The model under review builds one solid part; all positions refer to its coordinate system, in mm. Face numbers are marked on the shaded views. A direction names the side the tool comes from. Give positions to 0.01 mm unless a question says otherwise; leave off trailing zeros. Loops run counter-clockwise (first coordinate to the right, second up) from the corner with the lowest first, then second, coordinate; pieces in that order, holes last. Notation, with made-up numbers: (47, 54.25) - (91, 54.25) arc R20 cw to (91, 59.25) - close; hole circle Ø6 at (85, 5.5). An arc over 180 degrees is marked (long way). Answer as a JSON object with one key per item and string values.
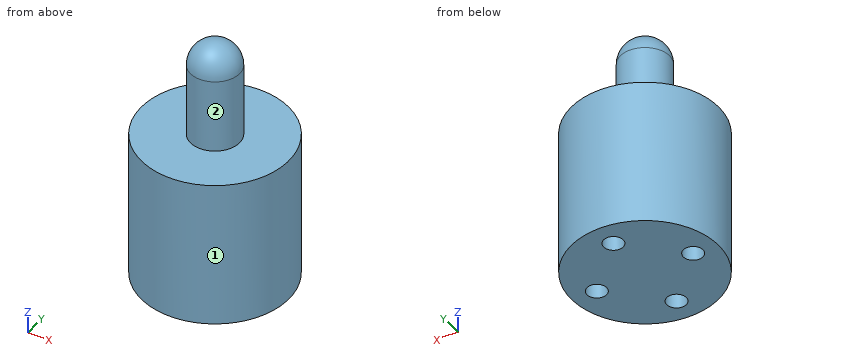
from build123d import *

# Parameters (mm, degrees)
F0_R     = 7.5
F1_DEPTH = 15
F2_R     = 1
F3_DEPTH = 5
F4_R     = 2.5
F5_DEPTH = 10
F6_R     = 2.5


with BuildPart() as f1:
    # F0 (on Top) → F1 (new body)
    with BuildSketch(Plane.XY):
        Circle(F0_R)
    extrude(amount=F1_DEPTH)

    # F2 (on face) → F3 (cut)
    with BuildSketch(Plane(origin=(0, 0, 0), x_dir=(1, 0, 0), z_dir=(0, 0, -1))):
        with Locations((0, 5)):
            Circle(F2_R)
        with Locations((-5, 0)):
            Circle(F2_R)
        with Locations((0, -5)):
            Circle(F2_R)
        with Locations((5, 0)):
            Circle(F2_R)
    extrude(amount=-F3_DEPTH, mode=Mode.SUBTRACT)

    # F4 (on face) → F5 (join)
    with BuildSketch(Plane.XY.offset(15)):
        Circle(F4_R)
    extrude(amount=F5_DEPTH)

    # F6
    f6_edges = [f1.edges().sort_by_distance(p)[0] for p in [
        (-2.5, 0, 25),
    ]]
    fillet(f6_edges, radius=F6_R)


solid = f1.part
Q1. Clearance check with flat-ended pins moving along their axes: pin 1 Ø6 at (x, z) = (-6, 7) entering from -Y; pin 2 Ø3 at (x, y) = (0, 5) entering from +Z; pin 3 Ø1.5 at (y, z) = (5, 13.5) entering from -X; pin 4 Ø2.5 at (x, y) = (-5, 0) entering from -Z. State where each tip first meets the part, or that it passes through.
Results:
{"pin 1": "stops at y = -6.87", "pin 2": "stops at z = 15", "pin 3": "stops at x = -6.18", "pin 4": "stops at z = 0"}
Q2. Consider section A-A, the plane z = 1.5. State the section outline as (x, y) points, plus the area to 3 significant figures.
Results:
{"outline": "circle Ø15 at (0, 0); hole circle Ø2 at (-5, 0); hole circle Ø2 at (0, -5); hole circle Ø2 at (0, 5); hole circle Ø2 at (5, 0)", "area": "164 mm^2"}
Q3. Consider section B-B, the plane x = 0. State the section outline as (y, z) points.
Results:
{"outline": "(-7.5, 0) - (-6, 0) - (-6, 5) - (-4, 5) - (-4, 0) - (4, 0) - (4, 5) - (6, 5) - (6, 0) - (7.5, 0) - (7.5, 15) - (2.5, 15) - (2.5, 22.5) arc R2.5 ccw to (-2.5, 22.5) - (-2.5, 15) - (-7.5, 15) - close"}
Q4. To check wall thickness, follow probe 1 along Y at (x, z) = (0, 2.7); probe 2 along Z at (x, y) = (5.5, -1); probe 3 along X at (y, z) = (5, 1.2). State the ranges of each line that lie inside material, in increasing order. Write a range as [from, to].
Results:
{"probe 1": "y = [-7.5, -6], [-4, 4], [6, 7.5]", "probe 2": "z = [0, 15]", "probe 3": "x = [-5.59, -1], [1, 5.59]"}
Q5. Consider section D-D, the plane y = -4.5. State the section outline as (x, z) points, plus the area to 3 significant figures.
Results:
{"outline": "(-6, 0) - (-0.87, 0) - (-0.87, 5) - (0.87, 5) - (0.87, 0) - (6, 0) - (6, 15) - (-6, 15) - close", "area": "171 mm^2"}
Q6. For the marked faces 1 and 2, list the 3-axis set-ups (+Z, -Z, +X, -X, +Y, -Y) from which the entire face can be reached by the end or side of a thin tool; tool diameter is ignored.
Results:
{"face 1": "+Z, -Z", "face 2": "+Z"}
